The model under review builds one solid part; all positions refer to its coordinate system, in mm. A direction names the side the tool comes from. Round coordinates to 2 decimals unless told otherwise and drop trailing zeros. Order: outer loops, then holes, each group sorted by start corner. A loop starts at its lowest first (then second) coordinate and runs counter-clockwise, first axis right, second up. Notation, with made-up numbers: (87, 67) -> (131, 67) arc R31 cw to (131, 93) -> close; hole circle Ø8 at (37.25, 23.5). An arc over 180 degrees is marked (long way). Return JSON: item names as keys, results as strings. Group by question number.
from build123d import *

# Parameters (mm, degrees)
BOSS_EXTRUDE1_DEPTH = 36.5125
SKETCH2_W           = 11.5
SKETCH2_H           = 8
BOSS_EXTRUDE2_DEPTH = 7.16


with BuildPart() as part:
    # Sketch1 → Boss-Extrude1 (new body)
    with BuildSketch(Plane(origin=(0, 0, 0), x_dir=(1, 0, 0), z_dir=(0, 1, 0))):
        with BuildLine():
            Line((-16.45, -69.245), (16.45, -69.245))
            Line((16.45, -69.245), (16.45, 69.245))
            ThreePointArc((16.45, 69.245), (13.512771736, 78.626231262), (5.75, 84.657332724))
            Line((5.75, 84.657332724), (5.75, 92.657332724))
            Line((5.75, 92.657332724), (-5.75, 92.657332724))
            Line((-5.75, 92.657332724), (-5.75, 84.657332724))
            ThreePointArc((-5.75, 84.657332724), (-13.512771736, 78.626231262), (-16.45, 69.245))
            Line((-16.45, 69.245), (-16.45, -69.245))
        make_face()
    extrude(amount=BOSS_EXTRUDE1_DEPTH)

    # Sketch2 → Boss-Extrude2 (add)
    with BuildSketch(Plane(origin=(0, 36.5125, 0), x_dir=(1, 0, 0), z_dir=(0, 1, 0))):
        with Locations((0, 88.657332724)):
            Rectangle(SKETCH2_W, SKETCH2_H)
    extrude(amount=BOSS_EXTRUDE2_DEPTH)


solid = part.part
Item 1: Insertion check: pin 1 Ø4 at (y, z) = (29, -87.5) entering from -X; pin 2 Ø2.5 at (y, z) = (29, -90.5) entering from +X; pin 3 Ø12 at (x, z) = (10, 13.5) entering from +Y. Each pin has a flat end and moves straight along its axis. Give the tip position at first contact, or say it passes through.
Item 2: Consider section C-C on z = 36.5. State the section outline as (x, y) points, plus the area to 3 significant figures.
Item 3: Wall thickness on line 1 along Y through (x, z) = (7, -9); line 2 along Z through (x, y) = (5, 40); line 3 along Z through (x, y) = (-9.5, 12) (3 decimals): over which ranges is each line inside the solid? List them lowest first.
Item 4: For faces 1 (the face through (-5.75, 22, -89)), 2 (the face through (5.75, 22, -89)), 3 (the face through (0, 36.512, -9)), list the 3-axis set-ups (+Z, -Z, +X, -X, +Y, -Y) from which the entire face can be reached by the end or side of a thin tool; tool diameter is ignored.
Item 5: Consider section D-D on z = -75. State the section outline as (x, y) points, plus the area to 3 significant figures.
Item 6: Consider section A-A on y = 30.5. State the section outline as (x, z) points (3 decimals).
Item 7: Consider section B-B on x = 1. State the section outline as (y, z) points (1 decimal), plus the area to 3 significant figures.
Values:
{
 "1": {"pin 1": "x = -5.75", "pin 2": "x = 5.75", "pin 3": "y = 36.51"},
 "2": {"outline": "(-16.45, 0) -> (16.45, 0) -> (16.45, 36.51) -> (-16.45, 36.51) -> close", "area": "1,200 mm^2"},
 "3": {"line 1": "0 to 36.51", "line 2": "-92.66 to -84.66", "line 3": "-82.675 to 69.245"},
 "4": {"face 1": "-Z, -X, +Y, -Y", "face 2": "-Z, +X, +Y, -Y", "face 3": "+Z, +X, -X, +Y"},
 "5": {"outline": "(-15.41, 0) -> (15.41, 0) -> (15.41, 36.51) -> (-15.41, 36.51) -> close", "area": "1,130 mm^2"},
 "6": {"outline": "(-16.45, -69.245) arc R16.45 ccw to (-5.75, -84.657) -> (-5.75, -92.657) -> (5.75, -92.657) -> (5.75, -84.657) arc R16.45 ccw to (16.45, -69.245) -> (16.45, 69.245) -> (-16.45, 69.245) -> close"},
 "7": {"outline": "(0, -92.7) -> (43.7, -92.7) -> (43.7, -84.7) -> (36.5, -84.7) -> (36.5, 69.2) -> (0, 69.2) -> close", "area": "5,970 mm^2"}
}
